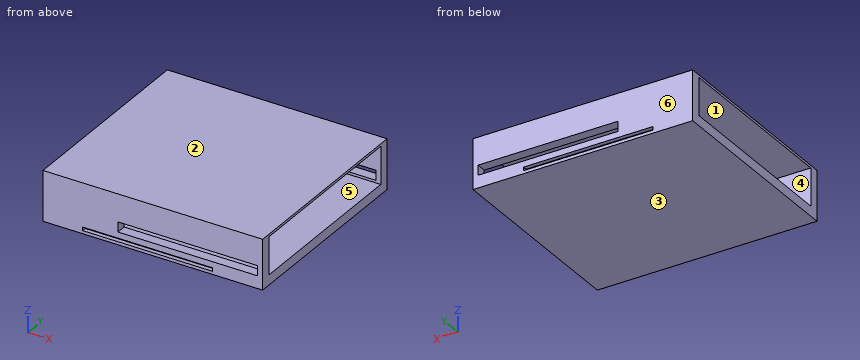
```python
from build123d import *

# Parameters (mm, degrees)
SKETCH1_W           = 440
SKETCH1_H           = 100
SKETCH1_W_2         = 280
SKETCH1_H_2         = 20
SKETCH1_W_3         = 260
SKETCH1_H_3         = 7
BOSS_EXTRUDE1_DEPTH = 20
SKETCH8_W           = 440
SKETCH8_H           = 5
BOSS_EXTRUDE2_DEPTH = 360
LPATTERN2_COUNT     = 2
LPATTERN2_PITCH     = 380
SKETCH10_W          = 440
SKETCH10_H          = 20
BOSS_EXTRUDE3_DEPTH = 360
SKETCH11_W          = 259.997812745
SKETCH11_H          = 3
CUT_EXTRUDE1_DEPTH  = 1.5
CUT_EXTRUDE2_DEPTH  = 1.5
SKETCH17_W          = 260
SKETCH17_H          = 3
CUT_EXTRUDE3_DEPTH  = 1.5
SKETCH18_W          = 260
SKETCH18_H          = 3
CUT_EXTRUDE4_DEPTH  = 1.5


with BuildPart() as part:
    # Sketch1 → Boss-Extrude1 (new body)
    with BuildSketch(Plane(origin=(0, 0, 0), x_dir=(1, 0, 0), z_dir=(0, 1, 0))):
        Rectangle(SKETCH1_W, SKETCH1_H)
        with Locations((70, 14.99604314)):
            Rectangle(SKETCH1_W_2, SKETCH1_H_2, mode=Mode.SUBTRACT)
        with Locations((-10.87698902, 40.5)):
            Rectangle(SKETCH1_W_3, SKETCH1_H_3, mode=Mode.SUBTRACT)
    boss_extrude1 = extrude(amount=BOSS_EXTRUDE1_DEPTH)

    # Sketch8 → Boss-Extrude2 (add)
    with BuildSketch(Plane.XZ):
        with Locations((0, 47.5)):
            Rectangle(SKETCH8_W, SKETCH8_H)
    extrude(amount=BOSS_EXTRUDE2_DEPTH)

    # LPattern2: Boss-Extrude1 ×2
    with Locations(*[(0, -i * LPATTERN2_PITCH, 0) for i in range(1, LPATTERN2_COUNT)]):
        add(boss_extrude1)

    # Sketch10 → Boss-Extrude3 (add)
    with BuildSketch(Plane.XZ):
        with Locations((0, -40)):
            Rectangle(SKETCH10_W, SKETCH10_H)
    extrude(amount=BOSS_EXTRUDE3_DEPTH)

    # Sketch11 → Cut-Extrude1 (cut)
    with BuildSketch(Plane(origin=(0, 0, -37), x_dir=(-1, 0, 0), z_dir=(0, 0, -1))):
        with Locations((10.878082647, 10)):
            Rectangle(SKETCH11_W, SKETCH11_H)
    extrude(amount=-CUT_EXTRUDE1_DEPTH, mode=Mode.SUBTRACT)

    # Sketch16 → Cut-Extrude2 (cut)
    with BuildSketch(Plane.XY.offset(-44)):
        Polygon((-140.87698902, 11.5), (119.12301098, 11.5), (119.12301098, 8.5), (-140.881315907, 8.5), align=None)
    extrude(amount=-CUT_EXTRUDE2_DEPTH, mode=Mode.SUBTRACT)

    # Sketch17 → Cut-Extrude3 (cut)
    with BuildSketch(Plane(origin=(0, 0, -37), x_dir=(-1, 0, 0), z_dir=(0, 0, -1))):
        with Locations((10.87698902, -370)):
            Rectangle(SKETCH17_W, SKETCH17_H)
    extrude(amount=-CUT_EXTRUDE3_DEPTH, mode=Mode.SUBTRACT)

    # Sketch18 → Cut-Extrude4 (cut)
    with BuildSketch(Plane.XY.offset(-44)):
        with Locations((-10.87698902, -370)):
            Rectangle(SKETCH18_W, SKETCH18_H)
    extrude(amount=-CUT_EXTRUDE4_DEPTH, mode=Mode.SUBTRACT)


solid = part.part
```
Geometry check sheet. Reference: the model listing, model coordinates, mm. Face numbers are marked on the shaded views. A direction names the side the tool comes from. Give positions to 0.01 mm unless a question says otherwise; leave off trailing zeros. Order: outer loops, then holes, each group sorted by start corner. A loop starts at its lowest first (then second) coordinate and runs counter-clockwise, first axis right, second up. Notation, with made-up numbers: (49, 10) - (88, 10) arc R17 ccw to (88, 26) - close; hole circle Ø5 at (87.5, 43.5). An arc over 180 degrees is marked (long way). Answer in a Markdown table with one row per item. Add a question column.
Q1. Cross-section at B-B, the plane y = -205.5. Enter the section's corners in (x, z), then the cut area to 3 significant figures.
Q2. Cross-section at A-A, the plane z = 12.5. Enter the section's corners in (x, y).
Q3. Tool access check on the marked faces 1 and 2. Record the directions out of +Z, -Z, +X, -X, +Y, -Y that give a thin tool (end or side, any length) a straight path to the whole face; none if there is none.
Q4. Mould release check, pull along Y, two halves, no side actions. Record for the marked faces 3, 4, 5 and 6: pulls with the +Y half, pulls with the -Y half, needs draft (parallel to the pull), parting line crosses it, or undercut.
Q5. Cross-section at D-D, the plane x = 132. Enter the section's corners in (y, z), then the cut area to 3 significant figures.
Q6. Material ranges on probe 1 along Y at (x, z) = (-87, -36.5); probe 2 along Y at (x, z) = (95, 19); probe 3 along Z at (x, y) = (175, -203), recorded low to high. Write a range as from..to.
Check values:
| question | item | result |
|---|---|---|
| 1 | outline | (-220, -50) - (220, -50) - (220, -30) - (-220, -30) - close; (-220, 45) - (220, 45) - (220, 50) - (-220, 50) - close |
| 1 | area | 11,000 mm^2 |
| 2 | outline | (-220, -380) - (220, -380) - (220, -360) - (-220, -360) - close; (-220, 0) - (220, 0) - (220, 20) - (-220, 20) - close |
| 3 | face 1 | +X, -X |
| 3 | face 2 | +Z, +X, -X, +Y, -Y |
| 4 | face 3 | needs draft |
| 4 | face 4 | undercut |
| 4 | face 5 | undercut |
| 4 | face 6 | pulls with the +Y half |
| 5 | outline | (-380, -50) - (20, -50) - (20, -25) - (0, -25) - (0, -30) - (-360, -30) - (-360, -25) - (-380, -25) - close; (-380, -5) - (-360, -5) - (-360, 45) - (0, 45) - (0, -5) - (20, -5) - (20, 50) - (-380, 50) - close |
| 5 | area | 12,200 mm^2 |
| 6 | probe 1 | y = -380..-371.5, -368.5..8.5, 11.5..20 |
| 6 | probe 2 | y = -380..-360, 0..20 |
| 6 | probe 3 | z = -50..-30, 45..50 |
